Geometry: final body of the model. Coordinates: model frame, mm. A direction names the side the tool comes from. Give positions to 0.01 mm unless a question says otherwise; leave off trailing zeros. Write each loop counter-clockwise with the first axis right and the second up, starting at its lowest first coordinate (ties: lowest second). Pieces come first, ordered by that corner, then holes. Notation, with made-up numbers: (69, 24) - (76, 24) arc R31 ccw to (76, 53) - close; hole circle Ø8 at (87.25, 31). An arc over 180 degrees is marked (long way). Return JSON: item names as keys, results as strings.
from build123d import *

# Parameters (mm, degrees)
BOSS_EXTRUDE1_DEPTH      = 5.5
SKETCH2_W                = 16.2
SKETCH2_H                = 1.35
CUT_EXTRUDE1_DEPTH       = 3
SKETCH5_W                = 18.2
SKETCH5_H                = 13.3
SKETCH5_W_2              = 9.8
SKETCH5_H_2              = 9.81
BOSS_EXTRUDE2_DEPTH      = 0.5
SKETCH6_W                = 11.107250644
SKETCH6_H                = 10.860006292
SKETCH6_W_2              = 8.9
SKETCH6_H_2              = 8.91
BOSS_EXTRUDE3_DEPTH      = 0.5
SKETCH7_W                = 16.2
SKETCH7_H                = 0.2
BOSS_EXTRUDE4_DEPTH      = 12.3
BOSS_EXTRUDE5_DEPTH      = 1.5
CUT_EXTRUDE7_DEPTH       = 19.035718964
CUT_EXTRUDE7_DEPTH_BACK  = 19.035718964
SKETCH10_R               = 1.2
SKETCH11_R               = 1.725
CUT_EXTRUDE11_DEPTH      = 10
CUT_EXTRUDE12_REACH      = 22.617
SKETCH17_W               = 9.8
SKETCH17_H               = 0.4
BOSS_EXTRUDE7_DEPTH      = 1.5
SKETCH19_W               = 8.904244722
SKETCH19_H               = 0.44
BOSS_EXTRUDE8_DEPTH      = 0.9
CUT_EXTRUDE13_DEPTH      = 1.5
CUT_EXTRUDE13_DEPTH_BACK = 1.5
SKETCH21_W               = 0.89
SKETCH21_H               = 1.9
BOSS_EXTRUDE9_START      = -10.25
SKETCH22_W               = 2.631722889
SKETCH22_H               = 2.55
SKETCH22_W_2             = 2.486658277
BOSS_EXTRUDE9_DEPTH      = 10.25
SKETCH23_W               = 3.968277111
SKETCH23_H               = 0.89
SKETCH23_W_2             = 4.113341723
BOSS_EXTRUDE11_DEPTH     = 2.05
CUT_EXTRUDE14_DEPTH      = 0.6


with BuildPart() as part:
    # Sketch1 → Boss-Extrude1 (new body)
    with BuildSketch(Plane(origin=(0, 0, 0), x_dir=(1, 0, 0), z_dir=(0, 1, 0))):
        Polygon((-11.065671851, -8.782275449), (-12.065671851, -8.782275449), (-12.065671851, 4.517724551), (6.134328149, 4.517724551), (6.134328149, -8.782275449), (5.134328149, -8.782275449), (5.134328149, 3.517724551), (-11.065671851, 3.517724551), align=None)
    extrude(amount=BOSS_EXTRUDE1_DEPTH)

    # Sketch2 → Cut-Extrude1 (cut)
    with BuildSketch(Plane(origin=(0, 0, -4.517724551), x_dir=(-1, 0, 0), z_dir=(0, 0, -1))):
        with Locations((2.965671851, 1.375)):
            Rectangle(SKETCH2_W, SKETCH2_H)
    extrude(amount=-CUT_EXTRUDE1_DEPTH, mode=Mode.SUBTRACT)

    # Sketch5 → Boss-Extrude2 (add)
    with BuildSketch(Plane(origin=(0, 5.5, 0), x_dir=(1, 0, 0), z_dir=(0, 1, 0))):
        with Locations((-2.965671851, -2.132275449)):
            Rectangle(SKETCH5_W, SKETCH5_H)
        with Locations((-2.965671851, -3.437275449)):
            Rectangle(SKETCH5_W_2, SKETCH5_H_2, mode=Mode.SUBTRACT)
    extrude(amount=BOSS_EXTRUDE2_DEPTH)

    # Sketch6 → Boss-Extrude3 (add)
    with BuildSketch(Plane.XZ.offset(-5.5)):
        with Locations((-2.90595545, 3.352272303)):
            Rectangle(SKETCH6_W, SKETCH6_H)
        with Locations((-2.965671851, 3.437275449)):
            Rectangle(SKETCH6_W_2, SKETCH6_H_2, mode=Mode.SUBTRACT)
    extrude(amount=BOSS_EXTRUDE3_DEPTH)

    # Sketch7 → Boss-Extrude4 (add)
    with BuildSketch(Plane.XY.offset(-3.517724551)):
        with Locations((-2.965671851, 2.85)):
            Rectangle(SKETCH7_W, SKETCH7_H)
    extrude(amount=BOSS_EXTRUDE4_DEPTH)

    # Sketch8 → Boss-Extrude5 (add)
    with BuildSketch(Plane(origin=(0, 0, 0), x_dir=(-1, 0, 0), z_dir=(0, -1, 0))):
        Polygon((11.065671851, -8.782275449), (11.065671851, 3.517724551), (11.065671851, 4.517724551), (12.065671851, 4.517724551), (14.565671851, 4.517724551), (14.565671851, -8.782275449), (12.065671851, -8.782275449), align=None)
        Polygon((-5.134328149, -8.782275449), (-5.134328149, 3.517724551), (-5.134328149, 4.517724551), (-6.134328149, 4.517724551), (-8.634328149, 4.517724551), (-8.634328149, -8.782275449), (-6.134328149, -8.782275449), align=None)
    extrude(amount=-BOSS_EXTRUDE5_DEPTH)

    # Sketch10 → Cut-Extrude7 (cut, two sides: drawn at the far end of the back side and taken through both)
    with BuildSketch(Plane(origin=(0, 0, 0), x_dir=(-1, 0, 0), z_dir=(0, -1, 0)).offset(-CUT_EXTRUDE7_DEPTH_BACK)):
        with Locations(Location((12.815671851, -6.587275449, 0), (0, 0, 90))):
            Circle(SKETCH10_R)
        with Locations(Location((12.815671851, -0.287275449, 0), (0, 0, 90))):
            Circle(SKETCH10_R)
        with Locations(Location((-6.884328149, -0.287275449, 0), (0, 0, 90))):
            Circle(SKETCH10_R)
        with Locations(Location((-6.884328149, -6.587275449, 0), (0, 0, 90))):
            Circle(SKETCH10_R)
    extrude(amount=CUT_EXTRUDE7_DEPTH + CUT_EXTRUDE7_DEPTH_BACK, mode=Mode.SUBTRACT)

    # Sketch11 → Cut-Extrude11 (cut)
    with BuildSketch(Plane(origin=(0, 1.5, 0), x_dir=(1, 0, 0), z_dir=(0, 1, 0))):
        with Locations((6.884328149, -0.287275449)):
            Circle(SKETCH11_R)
        with Locations((6.884328149, -6.587275449)):
            Circle(SKETCH11_R)
        with Locations((-12.815671851, -0.287275449)):
            Circle(SKETCH11_R)
        with Locations((-12.815671851, -6.587275449)):
            Circle(SKETCH11_R)
    extrude(amount=CUT_EXTRUDE11_DEPTH, mode=Mode.SUBTRACT)

    # Sketch17 → Cut-Extrude12 (cut, up to next)
    with BuildSketch(Plane.XY.offset(8.782275449), mode=Mode.PRIVATE) as cut_extrude12_sk1:
        with Locations((-2.965671851, 5.7)):
            Rectangle(SKETCH17_W, SKETCH17_H)
    cut_extrude12_tool1 = extrude(cut_extrude12_sk1.sketch, amount=-CUT_EXTRUDE12_REACH, mode=Mode.PRIVATE) & part.part
    add(cut_extrude12_tool1.solids().sort_by_distance((-2.965672, 5.7, 8.782275))[0], mode=Mode.SUBTRACT)

    # Sketch18 → Boss-Extrude7 (add)
    with BuildSketch(Plane(origin=(0, 6, 0), x_dir=(1, 0, 0), z_dir=(0, 1, 0))):
        Polygon((-7.419916573, -8.782275449), (-8.865671851, -8.782275449), (-8.865671851, 2.467724551), (-7.419916573, 2.467724551), (1.484328149, 2.467724551), (2.934328149, 2.467724551), (2.934328149, -8.782275449), (1.484328149, -8.782275449), (1.484328149, 1.017724551), (-7.419916573, 1.017724551), align=None)
    extrude(amount=BOSS_EXTRUDE7_DEPTH)

    # Sketch19 → Boss-Extrude8 (add)
    with BuildSketch(Plane(origin=(0, 6, 0), x_dir=(1, 0, 0), z_dir=(0, 1, 0))):
        with Locations((-2.967794212, -8.562275449)):
            Rectangle(SKETCH19_W, SKETCH19_H)
    extrude(amount=BOSS_EXTRUDE8_DEPTH)

    # Sketch21 → Cut-Extrude13 (cut, two sides: drawn at the far end of the back side and taken through both)
    with BuildSketch(Plane(origin=(-2.965671851, 0, 0), x_dir=(0, 0, -1), z_dir=(1, 0, 0)).offset(-CUT_EXTRUDE13_DEPTH_BACK)):
        with Locations((-8.337275449, 5.95)):
            Rectangle(SKETCH21_W, SKETCH21_H)
    extrude(amount=CUT_EXTRUDE13_DEPTH + CUT_EXTRUDE13_DEPTH_BACK, mode=Mode.SUBTRACT)

    # Sketch22 → Boss-Extrude9 (add)
    with BuildSketch(Plane.XY.offset(8.782275449).offset(BOSS_EXTRUDE9_START)):
        with Locations((-9.749810406, 4.225)):
            Rectangle(SKETCH22_W, SKETCH22_H)
        with Locations((3.89099901, 4.225)):
            Rectangle(SKETCH22_W_2, SKETCH22_H)
    extrude(amount=BOSS_EXTRUDE9_DEPTH)

    # Sketch23 → Boss-Extrude11 (add)
    with BuildSketch(Plane(origin=(0, 5, 0), x_dir=(1, 0, 0), z_dir=(0, 1, 0))):
        with Locations((-6.449810407, -8.337275449)):
            Rectangle(SKETCH23_W, SKETCH23_H)
        with Locations((0.590999011, -8.337275449)):
            Rectangle(SKETCH23_W_2, SKETCH23_H)
    extrude(amount=-BOSS_EXTRUDE11_DEPTH)

    # Sketch24 → Cut-Extrude14 (cut)
    with BuildSketch(Plane(origin=(0, 7.5, 0), x_dir=(1, 0, 0), z_dir=(0, 1, 0))):
        Polygon((-8.865671851, 1.017724551), (-8.865671851, -8.782275449), (-7.419916573, -8.782275449), (-7.419916573, 1.017724551), (1.484328149, 1.017724551), (1.484328149, -8.782275449), (2.934328149, -8.782275449), (2.934328149, 1.017724551), (2.934328149, 2.467724551), (1.484328149, 2.467724551), (-7.500141942, 2.467724551), (-8.865671851, 2.467724551), align=None)
    extrude(amount=-CUT_EXTRUDE14_DEPTH, mode=Mode.SUBTRACT)


solid = part.part
Q1. Section query A-A, the plane x = -9.5. Return the cut outline in (y, z), plus the area to 3 significant figures.
Answer key:
{"outline": "(0, -4.52) - (0.7, -4.52) - (0.7, -3.52) - (0, -3.52) - close; (2.05, -4.52) - (6, -4.52) - (6, 8.78) - (2.75, 8.78) - (2.75, -3.52) - (2.05, -3.52) - close; hole (2.95, -3.52) - (5.5, -3.52) - (5.5, -1.47) - (2.95, -1.47) - close", "area": "39.4 mm^2"}
Q2. Set-up query: faces 3 (the flat face through (-1.466, 4.2, 8.3)), 4 (the flat face through (-6, 4, 7.892)), 5 (the flat face through (-12.066, 4, -3)). Return all of +Z, -Z, +X, -X, +Y, -Y with unobstructed straight access to the full face (end or side cutting, diameter ignored); none if empty.
Answer key:
{"face 3": "+Z, +Y", "face 4": "none", "face 5": "+Z, -Z, -X, +Y"}
Q3. Material intervals for probe 1 along X at (y, z) = (1, 2); probe 2 along Z at (x, y) = (6.25, 0.5); probe 3 along Y at (x, z) = (-8.5, -4), sorted ascending. Write a range as [from, to].
Answer key:
{"probe 1": "x = [-14.57, -11.07], [5.13, 8.63]", "probe 2": "z = [-4.52, -0.73], [1.31, 5.57], [7.61, 8.78]", "probe 3": "y = [0, 0.7], [2.05, 6]"}
Q4. Pin query (flat end, axial travel): P1, Ø0.6, axis at y = 3.5, z = 5, coming from the +X side; P2, Ø4, axis at x = -9.5, z = 4, coming from the -Y side; P3, Ø0.5, axis at y = 6.5, z = 2, coming from the +X side; P4, Ø0.5, axis at x = -7, z = 8.5, coming from the -Y side. Return the tip coordinate at first contact, or that it passes through.
Answer key:
{"P1": "stops at x = 6.13", "P2": "stops at y = 0", "P3": "stops at x = 2.93", "P4": "stops at y = 2.75"}
Q5. Section query C-C, the plane y = 1.25. Return the cut outline in (x, z), plus the area to 3 significant figures.
Answer key:
{"outline": "(-14.57, -4.52) - (-11.07, -4.52) - (-11.07, 8.78) - (-14.57, 8.78) - close; (5.13, -4.52) - (8.63, -4.52) - (8.63, 8.78) - (5.13, 8.78) - close; hole circle Ø2.4 at (-12.82, 0.29); hole circle Ø2.4 at (-12.82, 6.59); hole circle Ø2.4 at (6.88, 0.29); hole circle Ø2.4 at (6.88, 6.59)", "area": "75.0 mm^2"}
Q6. Section query B-B, the plane x = -4. Return the cut outline in (y, z).
Answer key:
{"outline": "(0, -4.52) - (0.7, -4.52) - (0.7, -3.52) - (0, -3.52) - close; (2.05, -4.52) - (6, -4.52) - (6, -2.47) - (6.9, -2.47) - (6.9, -1.02) - (6, -1.02) - (6, -1.47) - (5.5, -1.47) - (5.5, -1.02) - (5, -1.02) - (5, -2.08) - (5.5, -2.08) - (5.5, -3.52) - (2.95, -3.52) - (2.95, 8.78) - (2.75, 8.78) - (2.75, -3.52) - (2.05, -3.52) - close"}
Q7. Mould query, pull axis Z, two halves, no side actions, for faces 1 (the flat face through (6.134, 4, -3)), 2 (the flat face through (-6.2, 6.4, 8.342)). Classes: pulls with the +Z half, pulls with the -Z half, needs draft (parallel to the pull), parting line crosses it, or undercut.
Answer key:
{"face 1": "needs draft", "face 2": "undercut"}
